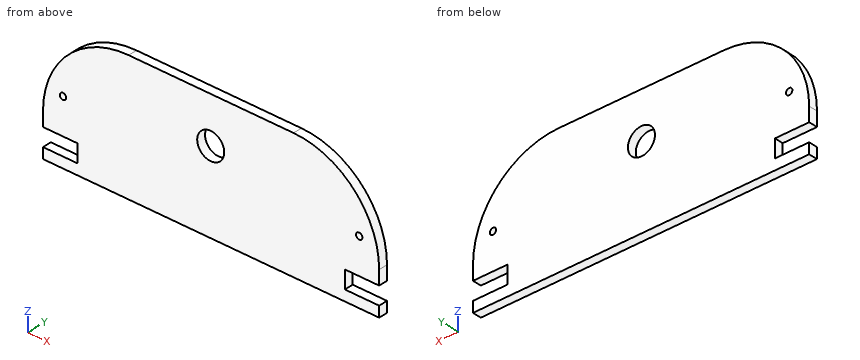
```python
from build123d import *

# Parameters (mm, degrees)
SKETCH1_W           = 119.634
SKETCH1_H           = 41.91
SKETCH1_R           = 4.8133
BOSS_EXTRUDE1_DEPTH = 3.175
SKETCH3_W           = 12.192
SKETCH3_H           = 6.35
CUT_EXTRUDE2_DEPTH  = 22.352
FILLET1_R           = 30.48
SKETCH4_W           = 119.634
SKETCH4_H           = 3.175
BOSS_EXTRUDE2_DEPTH = 3.81
SKETCH5_R           = 1.1303
CUT_EXTRUDE3_DEPTH  = 6.35
SKETCH6_R           = 1.1303
CUT_EXTRUDE4_DEPTH  = 6.35


with BuildPart() as part:
    # Sketch1 → Boss-Extrude1 (new body)
    with BuildSketch(Plane(origin=(0, 0, 0), x_dir=(1, 0, 0), z_dir=(0, 1, 0))):
        with Locations((59.817, 20.955)):
            Rectangle(SKETCH1_W, SKETCH1_H)
        with Locations(Location((59.69, 16.51, 0), (0, 0, 270))):
            Circle(SKETCH1_R, mode=Mode.SUBTRACT)
    extrude(amount=BOSS_EXTRUDE1_DEPTH)

    # Sketch3 → Cut-Extrude2 (cut)
    with BuildSketch(Plane(origin=(0, 3.175, 0), x_dir=(1, 0, 0), z_dir=(0, 1, 0))):
        with Locations((6.096, 38.735)):
            Rectangle(SKETCH3_W, SKETCH3_H)
        with Locations((113.538, 38.735)):
            Rectangle(SKETCH3_W, SKETCH3_H)
    extrude(amount=-CUT_EXTRUDE2_DEPTH, mode=Mode.SUBTRACT)

    # Fillet1
    fillet1_edges = [part.edges().sort_by_distance(p)[0] for p in [
        (119.634, 1.5875, 0),
        (0, 1.5875, 0),
    ]]
    fillet(fillet1_edges, radius=FILLET1_R)

    # Sketch4 → Boss-Extrude2 (add)
    with BuildSketch(Plane(origin=(0, 0, -41.91), x_dir=(-1, 0, 0), z_dir=(0, 0, -1))):
        with Locations((-59.817, 1.5875)):
            Rectangle(SKETCH4_W, SKETCH4_H)
    extrude(amount=BOSS_EXTRUDE2_DEPTH)

    # Sketch5 → Cut-Extrude3 (cut)
    with BuildSketch(Plane.XZ):
        with Locations(Location((7.112, -22.86, 0), (0, 0, 270))):
            Circle(SKETCH5_R)
    extrude(amount=-CUT_EXTRUDE3_DEPTH, mode=Mode.SUBTRACT)

    # Sketch6 → Cut-Extrude4 (cut)
    with BuildSketch(Plane.XZ):
        with Locations(Location((112.522, -22.86, 0), (0, 0, 270))):
            Circle(SKETCH6_R)
    extrude(amount=-CUT_EXTRUDE4_DEPTH, mode=Mode.SUBTRACT)


solid = part.part
```
Input: part model. Units: mm. Frame: model coordinates. Coordinates: 2 decimals unless noted, no trailing zeros. Loops run counter-clockwise (first coordinate to the right, second up) from the corner with the lowest first, then second, coordinate; pieces in that order, holes last. Notation, with made-up numbers: (49.5, 30) -> (92.5, 30) arc R32 cw to (92.5, 67) -> close; hole circle Ø6 at (26.5, 50.5). An arc over 180 degrees is marked (long way). Use a Markdown table: item, result.
1) Material intervals for line 1 along X through (y, z) = (2.35, -22.86); line 2 along X through (y, z) = (0.45, -23.5); line 3 along X through (y, z) = (1.6, -13), sorted ascending. Write a range as from..to.
Results found:
| item | result |
|---|---|
| line 1 | x = 0.97..5.98, 8.24..111.39, 113.65..118.67 |
| line 2 | x = 0.81..6.18, 8.04..111.59, 113.45..118.82 |
| line 3 | x = 5.51..56.4, 62.98..114.12 |
2) Cut plane A-A (x = 59.69). Return the cut outline in (y, z) (3 decimals), then the cut area to 3 significant figures.
Results found:
| item | result |
|---|---|
| outline | (0, -45.72) -> (3.175, -45.72) -> (3.175, -21.323) -> (0, -21.323) -> close; (0, -11.697) -> (3.175, -11.697) -> (3.175, 0) -> (0, 0) -> close |
| area | 115 mm2 |
3) Contact query for flat-ended pins moving along their axis: pin 1 (1.5 mm diameter, centred on x = 23, y = 1.5, fed in from +Z); pin 2 (1 mm diameter, centred on y = 1, z = -38.5, fed in from -X). Output: stop coordinate, or through.
Results found:
| item | result |
|---|---|
| pin 1 | stops at z = -0.75 |
| pin 2 | stops at x = 12.19 |
4) Cut plane B-B (z = -16.51). Return the cut outline in (x, y) (3 decimals).
Results found:
| item | result |
|---|---|
| outline | (3.39, 0) -> (54.877, 0) -> (54.877, 3.175) -> (3.39, 3.175) -> close; (64.503, 0) -> (116.244, 0) -> (116.244, 3.175) -> (64.503, 3.175) -> close |
5) Cut plane C-C (y = 0.6). Return the cut outline in (x, z).
Results found:
| item | result |
|---|---|
| outline | (0, -45.72) -> (119.63, -45.72) -> (119.63, -41.91) -> (107.44, -41.91) -> (107.44, -35.56) -> (119.63, -35.56) -> (119.63, -30.48) arc R30.48 ccw to (89.15, 0) -> (30.48, 0) arc R30.48 ccw to (0, -30.48) -> (0, -35.56) -> (12.19, -35.56) -> (12.19, -41.91) -> (0, -41.91) -> close; hole circle Ø2.26 at (7.11, -22.86); hole circle Ø9.63 at (59.69, -16.51); hole circle Ø2.26 at (112.52, -22.86) |
